Model file for the job. Use its own axes, mm. Face numbers are marked on the shaded views. A direction names the side the tool comes from. Round coordinates to 2 decimals unless told otherwise and drop trailing zeros. Order: outer loops, then holes, each group sorted by start corner. A loop starts at its lowest first (then second) coordinate and runs counter-clockwise, first axis right, second up. Notation, with made-up numbers: (-34.75, 0.25) -> (-11.75, 0.25) arc R32 cw to (-11.75, 28.25) -> close; hole circle Ø3 at (75, 55.5). An arc over 180 degrees is marked (long way). Put each result on its own line as item: value. Start each with the question number.
Q1. Cut at B-B, the plane z = 8. List the corners of the cut face in (x, y), and give its area (3 significant figures).
Q2. 3-axis set-ups, long thin cutter, end or side, ignore diameter. For the marked faces 1, 2, 3, 4 and 5: which of +Z, -Z, +X, -X, +Y, -Y reach the whole face in a straight line?
Q3. Cut at C-C, the plane x = -59.5. List the corners of the cut face in (y, z).
Q4. Cut at A-A, the plane y = -20.95. List the corners of the cut face in (x, z), and give its area (3 significant figures).
Q5. Cut at D-D, the plane z = 11.75. List the corners of the cut face in (x, y).
Q6. Flat gauge pins, fed straight in: P1, Ø5, axis at x = -44.21, y = -20.95, coming from the +Z side; P2, Ø3.5, axis at x = -42.5, z = 1, coming from the +Y side; P3, Ø7, axis at y = -8, z = 8.5, coming from the +X side. Where does each tip first touch, or does it go through?
Q7. Probe L1, parallel to X at y = -5.35, z = 8; L2, parallel to X at y = -20.95, z = 0.75; L3, parallel to X at y = -7.75, z = 0.25. List the from-to ranges inside material, lowest first.
from build123d import *

# Parameters (mm, degrees)
CROQUIS1_R              = 1.625
SALIENTE_EXTRUIR1_DEPTH = 3
CORTAR_EXTRUIR1_DEPTH   = 2
CROQUIS4_W              = 29.5
CROQUIS4_H              = 10.2
SALIENTE_EXTRUIR2_DEPTH = 3
SALIENTE_EXTRUIR3_DEPTH = 3
CROQUIS7_W              = 10
CROQUIS7_H              = 3
SALIENTE_EXTRUIR4_DEPTH = 5
CROQUIS9_W              = 10
CROQUIS9_H              = 3
SALIENTE_EXTRUIR5_DEPTH = 10
CROQUIS10_R             = 1.625
CORTAR_EXTRUIR2_DEPTH   = 3
CORTAR_EXTRUIR3_DEPTH   = 2
CORTAR_EXTRUIR4_START   = -10
CROQUIS12_W             = 3
CROQUIS12_H             = 5
CORTAR_EXTRUIR4_DEPTH   = 10


with BuildPart() as part:
    # Croquis1 → Saliente-Extruir1 (new body)
    with BuildSketch(Plane.XY):
        Polygon((-40.458841365, -24.7), (-77.458841365, -24.7), (-77.458841365, -14.45), (-47.958841365, -14.45), (-47.958841365, -17.2), (-40.458841365, -17.2), align=None)
        with Locations((-44.208841365, -20.95)):
            Circle(CROQUIS1_R, mode=Mode.SUBTRACT)
    extrude(amount=SALIENTE_EXTRUIR1_DEPTH)

    # Croquis2 → Cortar-Extruir1 (cut)
    with BuildSketch(Plane.XY.offset(3)):
        Polygon((-44.232492922, -17.739034302), (-46.977793452, -19.324034302), (-46.977793452, -22.494034302), (-44.232492922, -24.079034302), (-41.487192392, -22.494034302), (-41.487192392, -19.324034302), align=None)
    extrude(amount=-CORTAR_EXTRUIR1_DEPTH, mode=Mode.SUBTRACT)

    # Croquis4 → Saliente-Extruir2 (add)
    with BuildSketch(Plane(origin=(0, -14.45, 0), x_dir=(1, 0, 0), z_dir=(0, 1, 0))):
        with Locations((-62.708841365, 2.1)):
            Rectangle(CROQUIS4_W, CROQUIS4_H)
    extrude(amount=SALIENTE_EXTRUIR2_DEPTH)

    # Croquis6 → Saliente-Extruir3 (add)
    with BuildSketch(Plane.XY.offset(3)):
        Polygon((-62.708841365, -11.45), (-67.708841365, -11.45), (-67.708841365, -5), (-57.708841365, -5), (-57.708841365, -11.45), align=None)
    extrude(amount=-SALIENTE_EXTRUIR3_DEPTH)

    # Croquis7 → Saliente-Extruir4 (add)
    with BuildSketch(Plane(origin=(0, -5, 0), x_dir=(1, 0, 0), z_dir=(0, 1, 0))):
        with Locations((-62.708841365, -1.5)):
            Rectangle(CROQUIS7_W, CROQUIS7_H)
    extrude(amount=SALIENTE_EXTRUIR4_DEPTH)

    # Croquis9 → Saliente-Extruir5 (add)
    with BuildSketch(Plane.XY.offset(3)):
        with Locations((-62.708841365, -6.5)):
            Rectangle(CROQUIS9_W, CROQUIS9_H)
    extrude(amount=SALIENTE_EXTRUIR5_DEPTH)

    # Croquis10 → Cortar-Extruir2 (cut)
    with BuildSketch(Plane.XZ.offset(8)):
        with Locations(Location((-62.708841365, 8, 0), (0, 0, 270))):
            Circle(CROQUIS10_R)
    extrude(amount=-CORTAR_EXTRUIR2_DEPTH, mode=Mode.SUBTRACT)

    # Croquis11 → Cortar-Extruir3 (cut)
    with BuildSketch(Plane.XZ.offset(8)):
        Polygon((-62.708841365, 4.83), (-59.963540835, 6.415), (-59.963540835, 9.585), (-62.708841365, 11.17), (-65.454141895, 9.585), (-65.454141895, 6.415), align=None)
    extrude(amount=-CORTAR_EXTRUIR3_DEPTH, mode=Mode.SUBTRACT)

    # Croquis12 → Cortar-Extruir4 (cut)
    with BuildSketch(Plane(origin=(-57.708841365, 0, 0), x_dir=(0, 0, -1), z_dir=(1, 0, 0)).offset(CORTAR_EXTRUIR4_START)):
        with Locations((-1.5, -2.5)):
            Rectangle(CROQUIS12_W, CROQUIS12_H)
    extrude(amount=CORTAR_EXTRUIR4_DEPTH, mode=Mode.SUBTRACT)


solid = part.part
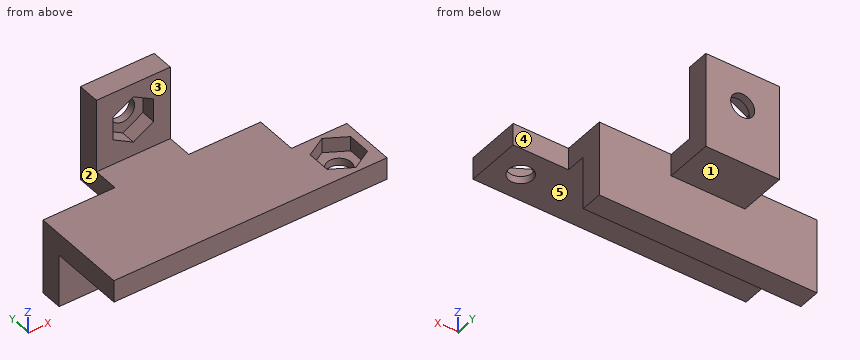
Ans:
1. outline: (-67.71, -8) -> (-65.45, -8) -> (-65.45, -6) -> (-64.33, -6) -> (-64.33, -5) -> (-67.71, -5) -> close; (-61.08, -6) -> (-59.96, -6) -> (-59.96, -8) -> (-57.71, -8) -> (-57.71, -5) -> (-61.08, -5) -> close
1. area: 15.8 mm^2
2. face 1: -Z, +X, -X, +Y
2. face 2: +Z, -Z, -X, +Y
2. face 3: +Z, +X, -X, -Y
2. face 4: +Z, -Z, +X, +Y
2. face 5: -Z, +X, -X, -Y
3. outline: (-24.7, 0) -> (-14.45, 0) -> (-14.45, -7.2) -> (-11.45, -7.2) -> (-11.45, 0) -> (-5, 0) -> (-5, 13) -> (-8, 13) -> (-8, 3) -> (-24.7, 3) -> close
4. outline: (-77.46, 0) -> (-45.83, 0) -> (-45.83, 1) -> (-46.98, 1) -> (-46.98, 3) -> (-77.46, 3) -> close; (-42.58, 0) -> (-40.46, 0) -> (-40.46, 3) -> (-41.49, 3) -> (-41.49, 1) -> (-42.58, 1) -> close
4. area: 96.8 mm^2
5. outline: (-67.71, -8) -> (-57.71, -8) -> (-57.71, -5) -> (-67.71, -5) -> close
6. P1: stops at z = 1
6. P2: stops at y = -17.2
6. P3: stops at x = -57.71
7. L1: x = -67.71 to -64.33, -61.08 to -57.71
7. L2: x = -77.46 to -45.83, -42.58 to -40.46
7. L3: x = -67.71 to -57.71
